Source: CAD feature listing. Evaluate the final solid. Frame: model axes, mm. Face numbers are marked on the shaded views. Round coordinates to 2 decimals unless told otherwise and drop trailing zeros. Loops run counter-clockwise (first coordinate to the right, second up) from the corner with the lowest first, then second, coordinate; pieces in that order, holes last.
(1) Section A-A, the plane z = -0.3. Return the cut outline in (x, y).
(2) Material intervals for probe 1 along X at (y, z) = (1.6, 0.8); probe 2 along Z at (x, y) = (6, 1.8); probe 3 along Z at (x, y) = (-7.75, 1.5), sorted ascending.
(3) First-contact query: pin 1 Ø1 at (x, y) = (2.5, -1.5) entering from -Z. Flat tip, straight axial feed; report the tip coordinate or a pass-through.
(4) Mould query, pull axis Y, two halves, no side actions, for the marked faces 1 and 2. Classes: pulls with the +Y half, pulls with the -Y half, needs draft (parallel to the pull), parting line crosses it, or undercut.
(5) Section B-B, the plane x = 5.25. Return the cut outline in (y, z), plus the area to 3 significant figures.
(6) Section C-C, the plane y = 1.3. Return the cut outline in (x, z).
```python
from build123d import *

# Parameters (mm, degrees)
SKETCH1_R           = 2
BOSS_EXTRUDE1_DEPTH = 9.75
SKETCH2_W           = 0.64
SKETCH2_H           = 0.4


with BuildPart() as part:
    # Sketch1 → Boss-Extrude1 (new, symmetric)
    with BuildSketch(Plane(origin=(0, 0, 0), x_dir=(0, 0, -1), z_dir=(1, 0, 0))):
        Circle(SKETCH1_R)
    extrude(amount=BOSS_EXTRUDE1_DEPTH, both=True)

    # Sketch2 → Cut-Revolve1 (revolve, cut)
    with BuildSketch(Plane(origin=(0, 0, 0), x_dir=(1, 0, 0), z_dir=(0, 1, 0)), mode=Mode.PRIVATE) as cut_revolve1_sk:
        with Locations((-8.42, 1.8)):
            Rectangle(SKETCH2_W, SKETCH2_H)
    cut_revolve1 = revolve(cut_revolve1_sk.sketch.rotate(Axis((-10.725, 0, 0), (1, 0, 0)), 180), axis=Axis((-10.725, 0, 0), (1, 0, 0)), mode=Mode.SUBTRACT)

    # Mirror1: Cut-Revolve1 across plane
    add(cut_revolve1.mirror(Plane(origin=(0, 0, 0), x_dir=(0, 0, 1), z_dir=(1, 0, 0))), mode=Mode.SUBTRACT)


solid = part.part
```
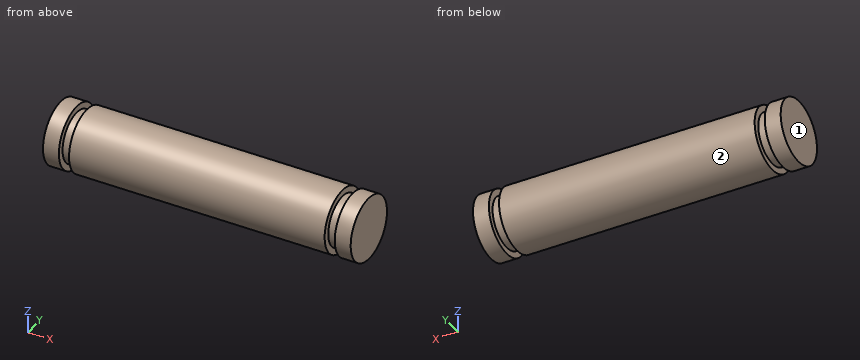
Output values:
1. outline: (-9.75, -1.98) - (-8.74, -1.98) - (-8.74, -1.57) - (-8.1, -1.57) - (-8.1, -1.98) - (8.1, -1.98) - (8.1, -1.57) - (8.74, -1.57) - (8.74, -1.98) - (9.75, -1.98) - (9.75, 1.98) - (8.74, 1.98) - (8.74, 1.57) - (8.1, 1.57) - (8.1, 1.98) - (-8.1, 1.98) - (-8.1, 1.57) - (-8.74, 1.57) - (-8.74, 1.98) - (-9.75, 1.98) - close
2. probe 1: x = -9.75 to -8.74, -8.1 to 8.1, 8.74 to 9.75
2. probe 2: z = -0.87 to 0.87
2. probe 3: z = -1.32 to 1.32
3. pin 1: stops at z = -1.73
4. face 1: needs draft
4. face 2: parting line crosses it
5. outline: circle Ø4 at (0, 0)
5. area: 12.6 mm2
6. outline: (-9.75, -1.52) - (-8.74, -1.52) - (-8.74, -0.93) - (-8.1, -0.93) - (-8.1, -1.52) - (8.1, -1.52) - (8.1, -0.93) - (8.74, -0.93) - (8.74, -1.52) - (9.75, -1.52) - (9.75, 1.52) - (8.74, 1.52) - (8.74, 0.93) - (8.1, 0.93) - (8.1, 1.52) - (-8.1, 1.52) - (-8.1, 0.93) - (-8.74, 0.93) - (-8.74, 1.52) - (-9.75, 1.52) - close
